```python
from build123d import *

# Parameters (mm, degrees)
SKETCH067_W     = 20
SKETCH067_H     = 20
PAD025_DEPTH    = 9
SKETCH061_R     = 7
PAD024_DEPTH    = 10
POCKET040_DEPTH = 8
SKETCH063_W     = 8.75
SKETCH063_H     = 5.2
POCKET036_DEPTH = 1
SKETCH060_R     = 3.7
POCKET035_DEPTH = 3
SKETCH059_R     = 1.675
POCKET039_DEPTH = 5
SKETCH068_R     = 16.754851
SKETCH068_R_2   = 9.771783
POCKET041_DEPTH = 20
SKETCH062_R     = 1.7
POCKET042_DEPTH = 20
FILLET008_R     = 1.2
POCKET043_DEPTH = 5.2


with BuildPart() as part:
    # Sketch067 → Pad025 (new body)
    with BuildSketch(Plane.XZ):
        with Locations((-19.773271, -18.660706)):
            Rectangle(SKETCH067_W, SKETCH067_H)
    extrude(amount=PAD025_DEPTH)

    # Sketch061 (on Face6 of Pad025) → Pad024 (join)
    with BuildSketch(Plane.XZ.offset(9)):
        with Locations((-19.773271, -18.660706)):
            Circle(SKETCH061_R)
    extrude(amount=PAD024_DEPTH)

    # Sketch065 (on Face8 of Pad024) → Pocket040 (cut)
    with BuildSketch(Plane.XZ.offset(19)):
        with BuildLine():
            Line((-17.123271, -18.660706), (-17.123271, -31.745383))
            Line((-17.123271, -31.745383), (-22.423271, -31.745383))
            Line((-22.423271, -31.745383), (-22.423271, -18.660706))
            ThreePointArc((-17.123271, -18.660706), (-19.773271, -16.010706), (-22.423271, -18.660706))
        make_face()
    extrude(amount=-POCKET040_DEPTH, mode=Mode.SUBTRACT)

    # Sketch063 (on Face6 of Pocket040) → Pocket036 (cut)
    with BuildSketch(Plane(origin=(0, 0, -28.660706), x_dir=(1, 0, 0), z_dir=(0, 0, -1))):
        with Locations((-19.773271, 11.6)):
            Rectangle(SKETCH063_W, SKETCH063_H)
    extrude(amount=-POCKET036_DEPTH, mode=Mode.SUBTRACT)

    # Sketch060 (on Face4 of Pocket036) → Pocket035 (cut)
    with BuildSketch(Plane(origin=(0, 0, 0), x_dir=(1, 0, 0), z_dir=(0, 1, 0))):
        with Locations((-19.773271, 18.660706)):
            Circle(SKETCH060_R)
    extrude(amount=-POCKET035_DEPTH, mode=Mode.SUBTRACT)

    # Sketch059 (on Face11 of Pocket035) → Pocket039 (cut)
    with BuildSketch(Plane.XZ.offset(19)):
        with Locations((-19.773271, -18.660706)):
            Circle(SKETCH059_R)
    extrude(amount=-POCKET039_DEPTH, mode=Mode.SUBTRACT)

    # Sketch068 (on Face4 of Pocket039) → Pocket041 (cut)
    with BuildSketch(Plane(origin=(0, 0, 0), x_dir=(1, 0, 0), z_dir=(0, 1, 0))):
        with Locations((-19.773271, 18.660706)):
            Circle(SKETCH068_R)
        with Locations((-19.773271, 18.660706)):
            Circle(SKETCH068_R_2, mode=Mode.SUBTRACT)
    extrude(amount=-POCKET041_DEPTH, mode=Mode.SUBTRACT)

    # Sketch062 → Pocket042 (cut)
    with BuildSketch(Plane(origin=(0, -3, 0), x_dir=(1, 0, 0), z_dir=(0, 1, 0))):
        with Locations((-19.773271, 18.660706)):
            Circle(SKETCH062_R)
    extrude(amount=-POCKET042_DEPTH, mode=Mode.SUBTRACT)

    # Fillet008
    fillet008_edges = [part.edges().sort_by_distance(p)[0] for p in [
        (-19.773271, -9, -27.660706),
        (-25.172051, -9, -10.515712),
        (-11.628277, -9, -24.059485),
        (-26.773271, -9, -18.660706),
        (-29.545054, 0, -18.660706),
        (-23.473271, 0, -18.660706),
    ]]
    fillet(fillet008_edges, radius=FILLET008_R)

    # Sketch064 → Pocket043 (cut)
    with BuildSketch(Plane.XZ.offset(14.2)):
        with BuildLine():
            ThreePointArc((-15.373271, -18.660706), (-19.773271, -14.260706), (-24.173271, -18.660706))
            Line((-24.173271, -18.660706), (-24.173271, -31.35503))
            Line((-24.173271, -31.35503), (-15.373271, -31.35503))
            Line((-15.373271, -18.660706), (-15.373271, -31.35503))
        make_face()
    extrude(amount=-POCKET043_DEPTH, mode=Mode.SUBTRACT)


solid = part.part
```
Verification items for the finished model (mm, model axes). A direction names the side the tool comes from. Round coordinates to 2 decimals unless told otherwise and drop trailing zeros. Write each loop counter-clockwise with the first axis right and the second up, starting at its lowest first coordinate (ties: lowest second). Pieces come first, ordered by that corner, then holes.
1. Access from +Z, -Z, +X, -X, +Y, -Y to the whole of each face (thin tool, end or side, straight path). Record for faces 1 (the flat face through (-17.123, -17, -22)), 2 (the cylindrical face through (-19.68, -11.64, -14.26)), 3 (the flat face through (-18, -3, -18)).
2. Section check C-C on y = -2.5. Enter the section's corners in (x, z).
3. Section check D-D on y = -10.75. Enter the section's corners in (x, z), plus the area to 3 significant figures.
4. Section check A-A on y = -7.5. Enter the section's corners in (x, z).
5. Draft check along X on faces 4 (the flat face through (-16.9, -14.2, -19.6)), 5 (the cylindrical face through (-21.05, -4.45, -28.35)), 6 (the flat face through (-20, -19, -15)). Enter one of: +X half, -X half, draft (parallel to the pull), parting line (faces both ways), or undercut.
6. Section check B-B on y = -14.5. Enter the section's corners in (x, z).
7. Scan lines: L1, parallel to X at y = -16.25, z = -25; L2, parallel to Y at x = -25.5, z = -12.5; L3, parallel to X at y = -10.25, z = -16.25. Record each from-to range of solid material in increasing order.
8. Gauge pin test, flat ends, axial feed: P1, Ø4, axis at x = -19.77, z = -18.66, coming from the +Y side; P2, Ø8, axis at x = -14.5, y = -7.5, coming from the -Z side; P3, Ø4, axis at y = -17.5, z = -20.5, coming from the -X side. Record the tip position at first contact, or that the pin passes through.
Answer:
1. face 1: -Z, -Y
1. face 2: -Z
1. face 3: +Y
2. outline: circle Ø19.54 at (-19.77, -18.66); hole circle Ø7.4 at (-19.77, -18.66)
3. outline: (-24.17, -24.1) - (-24.17, -18.66) arc R4.4 cw to (-15.37, -18.66) - (-15.37, -24.1) arc R7 ccw (long way) to start
3. area: 66.3 mm2
4. outline: circle Ø19.54 at (-19.77, -18.66); hole circle Ø3.4 at (-19.77, -18.66)
5. face 4: undercut
5. face 5: parting line
5. face 6: draft
6. outline: (-22.42, -25.14) - (-22.42, -18.66) arc R2.65 cw to (-17.12, -18.66) - (-17.12, -25.14) arc R7 ccw (long way) to start
7. L1: x = -22.74 to -22.42, -17.12 to -16.8
7. L2: y = -9 to 0
7. L3: x = -26.35 to -23.45, -16.09 to -13.2
8. P1: stops at y = -3
8. P2: stops at z = -28.35
8. P3: stops at x = -26.77
